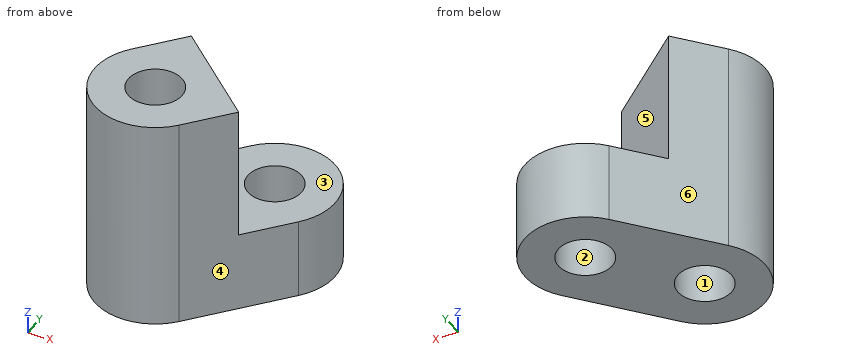
```python
from build123d import *

# Parameters (mm, degrees)
SKETCH3_R           = 1
BOSS_EXTRUDE1_DEPTH = 8
CUT_EXTRUDE1_START  = -5
CUT_EXTRUDE1_DEPTH  = 5


with BuildPart() as part:
    # Sketch3 → Boss-Extrude1 (new body)
    with BuildSketch(Plane(origin=(0, 0, 0), x_dir=(0, 1, 0), z_dir=(0, 0, 1))):
        with BuildLine():
            Line((-9.209045769, 12.846172912), (-12.389045769, 15.561172912))
            ThreePointArc((-12.389045769, 15.561172912), (-15.561172912, 15.310954231), (-15.310954231, 12.138827088))
            Line((-15.310954231, 12.138827088), (-12.130954231, 9.423827088))
            ThreePointArc((-12.130954231, 9.423827088), (-8.958827088, 9.674045769), (-9.209045769, 12.846172912))
        make_face()
        with Locations(Location((-13.85, 13.85, 0), (0, 0, 270))):
            Circle(SKETCH3_R, mode=Mode.SUBTRACT)
        with Locations(Location((-10.67, 11.135, 0), (0, 0, 270))):
            Circle(SKETCH3_R, mode=Mode.SUBTRACT)
    extrude(amount=BOSS_EXTRUDE1_DEPTH)

    # Sketch4 → Cut-Extrude1 (cut)
    with BuildSketch(Plane.XY.offset(8).offset(CUT_EXTRUDE1_START)):
        with BuildLine():
            Line((-12.846172912, -9.209045769), (-14.203672912, -10.799045769))
            Line((-14.203672912, -10.799045769), (-10.781327088, -13.720954231))
            Line((-10.781327088, -13.720954231), (-9.423827088, -12.130954231))
            ThreePointArc((-9.423827088, -12.130954231), (-9.674045769, -8.958827088), (-12.846172912, -9.209045769))
        make_face()
    extrude(amount=CUT_EXTRUDE1_DEPTH, mode=Mode.SUBTRACT)


solid = part.part
```
Geometry check sheet. Reference: the model listing, model coordinates, mm. Face numbers are marked on the shaded views. A direction names the side the tool comes from. Give positions to 0.01 mm unless a question says otherwise; leave off trailing zeros. Order: outer loops, then holes, each group sorted by start corner. A loop starts at its lowest first (then second) coordinate and runs counter-clockwise, first axis right, second up. Notation, with made-up numbers: (10.5, 14.25) - (59.5, 14.25) arc R21 ccw to (59.5, 18.25) - close; hole circle Ø2 at (20.25, 63.25). An arc over 180 degrees is marked (long way). Write item = value, one per line. Start each with the question number.
1) Draft check along Y on the marked faces 1, 2, 3 and 4. Enter one of: released by +Y, released by -Y, zero draft, split by the parting line, or undercut.
2) Scan lines: L1, parallel to X at y = -13.25, z = 5; L2, parallel to X at y = -14.25, z = 3.75; L3, parallel to Z at x = -13.5, y = -10.25. Record each from-to range of solid material in increasing order.
3) Access from +Z, -Z, +X, -X, +Y, -Y to the whole of each face (thin tool, end or side, straight path). Record for the marked faces 5 and 6.
4) Section check C-C (x = -13.85). Enter the section's corners in (y, z).
5) Section check B-B (y = -13). Enter the section's corners in (x, z), then the cut area to 3 significant figures.
6) Gauge pin test, flat ends, axial feed: pin 1 Ø1.5 at (x, z) = (-15, 4) entering from +Y; pin 2 Ø1 at (x, z) = (-10, 1.5) entering from -Y; pin 3 Ø3 at (x, y) = (-11.135, -10.67) entering from +Z. Record the tip position at first contact, or that the pin passes through.
7) Section check D-D (y = -13.85). Enter the section's corners in (x, z), then the cut area to 3 significant figures.
Geometry check:
q1.face_1 = undercut
q1.face_2 = undercut
q1.face_3 = zero draft
q1.face_4 = released by -Y
q2.L1 = -16.02 to -14.65, -13.05 to -11.33
q2.L2 = -16.06 to -14.77, -12.93 to -11.23
q2.L3 = 0 to 3
q3.face_5 = +Z, +X, +Y
q3.face_6 = +Z, -Z, -X, +Y
q4.outline = (-16.1, 0) - (-14.85, 0) - (-14.85, 8) - (-16.1, 8) - close; (-12.85, 0) - (-10.38, 0) - (-10.38, 3) - (-11.1, 3) - (-11.1, 8) - (-12.85, 8) - close
q5.outline = (-15.93, 0) - (-14.38, 0) - (-14.38, 8) - (-15.93, 8) - close; (-13.32, 0) - (-10.17, 0) - (-10.17, 3) - (-11.63, 3) - (-11.63, 8) - (-13.32, 8) - close
q5.area = 30.4 mm2
q6.pin_1 = -10.85
q6.pin_2 = -13.39
q6.pin_3 = 3
q7.outline = (-16.1, 0) - (-14.85, 0) - (-14.85, 8) - (-16.1, 8) - close; (-12.85, 0) - (-10.89, 0) - (-10.89, 8) - (-12.85, 8) - close
q7.area = 25.7 mm2
